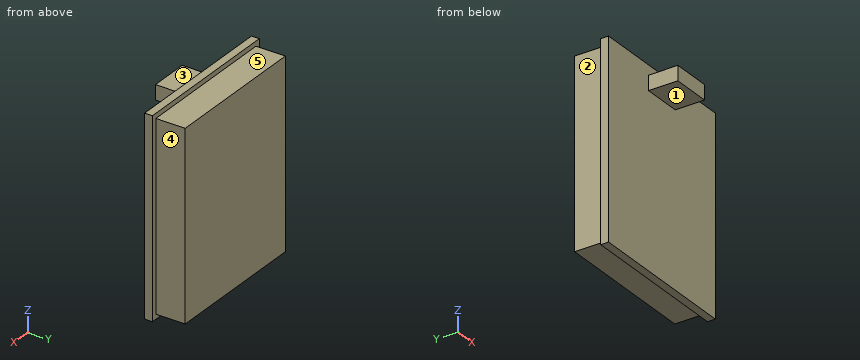
from build123d import *

# Parameters (mm, degrees)
SKETCH1_W           = 32
SKETCH1_H           = 40
BOSS_EXTRUDE1_DEPTH = 1.6
SKETCH2_W           = 30
SKETCH2_H           = 38
BOSS_EXTRUDE2_DEPTH = 6
SKETCH3_W           = 8
SKETCH3_H           = 3
BOSS_EXTRUDE3_DEPTH = 6


with BuildPart() as part:
    # Sketch1 → Boss-Extrude1 (new body)
    with BuildSketch(Plane(origin=(0, 0, 0), x_dir=(1, 0, 0), z_dir=(0, 1, 0))):
        with Locations((16, 20)):
            Rectangle(SKETCH1_W, SKETCH1_H)
    extrude(amount=BOSS_EXTRUDE1_DEPTH)

    # Sketch2 → Boss-Extrude2 (add)
    with BuildSketch(Plane(origin=(0, 1.6, 0), x_dir=(1, 0, 0), z_dir=(0, 1, 0))):
        with Locations((16, 20)):
            Rectangle(SKETCH2_W, SKETCH2_H)
    extrude(amount=BOSS_EXTRUDE2_DEPTH)

    # Sketch3 → Boss-Extrude3 (add)
    with BuildSketch(Plane.XZ):
        with Locations((16, -3.5)):
            Rectangle(SKETCH3_W, SKETCH3_H)
    extrude(amount=BOSS_EXTRUDE3_DEPTH)


solid = part.part
Can you work these out from the model? Positions are in its coordinate system, mm. Face numbers are marked on the shaded views. A direction names the side the tool comes from. Give positions to 0.01 mm unless a question says otherwise; leave off trailing zeros. Write each loop counter-clockwise with the first axis right and the second up, starting at its lowest first coordinate (ties: lowest second). Pieces come first, ordered by that corner, then holes. Notation, with made-up numbers: M 14.25,-2.5 L 43.25,-2.5 A27 ccw 43.25,22.5 Z; hole C 72.25,49.5 d6. An arc over 180 degrees is marked long. Answer in a Markdown table with one row per item. Add a question column.
Item 1: Please list where these lines run through material, in increasing order: L1, parallel to Y at x = 14.5, z = -27.5; L2, parallel to X at y = 6.25, z = -16; L3, parallel to Z at x = 13, y = -0.25.
Item 2: Imagine slicing it at D-D, the plane x = 19. Write out the boundary of the cut face in (y, z).
Item 3: On a 3-axis mill with a long thin cutter (end or side, diameter ignored), from which of +Z, -Z, +X, -X, +Y, -Y can I reach the whole of each face in a straight line? I mean the marked faces 1, 2, 3, 4 and 5. Say none if no direction works.
Item 4: Imagine slicing it at C-C, the plane y = 4.5. Write out the boundary of the cut face in (x, z), plus the area to 3 significant figures.
Item 5: For pin 1 Ø6.5 at (x, y) = (14, -3) entering from -Z; pin 2 Ø3 at (y, z) = (6, -25) entering from -X; pin 3 Ø9.5 at (x, z) = (8.5, -12.5) entering from -Y; pin 4 Ø3 at (x, y) = (14, 5.5) entering from +Z, each with a flat end and sliding along its axis, tell me the tip position at first contact or that it passes through.
Item 6: Imagine slicing it at A-A, the plane x = 27. Write out the boundary of the cut face in (y, z), plus the area to 3 significant figures.
Item 7: Imagine slicing it at B-B, the plane z = -12. Write out the boundary of the cut face in (x, y).
Evaluation:
| question | item | result |
|---|---|---|
| 1 | L1 | y = 0 to 7.6 |
| 1 | L2 | x = 1 to 31 |
| 1 | L3 | z = -5 to -2 |
| 2 | outline | M -6,-5 L 0,-5 L 0,-40 L 1.6,-40 L 1.6,-39 L 7.6,-39 L 7.6,-1 L 1.6,-1 L 1.6,0 L 0,0 L 0,-2 L -6,-2 Z |
| 3 | face 1 | -Z, +X, -X, -Y |
| 3 | face 2 | +Z, -Z, -X, +Y |
| 3 | face 3 | +Z, +X, -X, -Y |
| 3 | face 4 | +Z, -Z, +X, +Y |
| 3 | face 5 | +Z, +X, -X, +Y |
| 4 | outline | M 1,-39 L 31,-39 L 31,-1 L 1,-1 Z |
| 4 | area | 1,140 mm² |
| 5 | pin 1 | stops at z = -40 |
| 5 | pin 2 | stops at x = 1 |
| 5 | pin 3 | stops at y = 0 |
| 5 | pin 4 | stops at z = -1 |
| 6 | outline | M 0,-40 L 1.6,-40 L 1.6,-39 L 7.6,-39 L 7.6,-1 L 1.6,-1 L 1.6,0 L 0,0 Z |
| 6 | area | 292 mm² |
| 7 | outline | M 0,0 L 32,0 L 32,1.6 L 31,1.6 L 31,7.6 L 1,7.6 L 1,1.6 L 0,1.6 Z |
